Design review of the part built by this model. Coordinates are the model's own, in mm. A direction names the side the tool comes from. Give positions to 0.01 mm unless a question says otherwise; leave off trailing zeros. Loops run counter-clockwise (first coordinate to the right, second up) from the corner with the lowest first, then second, coordinate; pieces in that order, holes last. Notation, with made-up numbers: (-0.5, 4) - (46.5, 4) arc R23 cw to (46.5, 32) - close; hole circle Ø10 at (-36.5, 72.5). An arc over 180 degrees is marked (long way). One line per item, written item: value. Start each with the question number.
```python
from build123d import *

# Parameters (mm, degrees)
F0_W     = 46.54321
F0_H     = 54.078784
F1_DEPTH = 25.4
F2_R     = 6.959459
F2_R_2   = 6.442665
F3_DEPTH = 50.8
F4_R     = 2.356005
F5_DEPTH = 50.8


with BuildPart() as f1:
    # F0 (on Front) → F1 (new body)
    with BuildSketch(Plane.XZ):
        Rectangle(F0_W, F0_H)
    extrude(amount=F1_DEPTH)

    # F2 (on face) → F3 (cut)
    with BuildSketch(Plane.XY.offset(27.039392)):
        with Locations((-11.081717, -13.741329)):
            Circle(F2_R)
        with Locations((10.416814, -13.741329)):
            Circle(F2_R_2)
    extrude(amount=-F3_DEPTH, mode=Mode.SUBTRACT)

    # F4 (on face) → F5 (join)
    with BuildSketch(Plane.XZ.offset(25.4)):
        with Locations((0, 22.828339)):
            Circle(F4_R)
    extrude(amount=F5_DEPTH)


solid = f1.part
```
(1) Machinability: for faces 1 (the cylindrical face through (-12.59, -20.535, 1.995)), 2 (the flat face through (0, 0, 0)), 3 (the cylindrical face through (-0.307, -50.444, 25.164)), which of the approach directions +Z, -Z, +X, -X, +Y, -Y give a long, thin tool a straight path to every point of the face, cutting with its end or side? Answer none if there is none.
(2) Take a section at D-D on x = -6. State the section outline as (y, z) points.
(3) To check wall thickness, follow L1, parallel to X at y = -19, z = -8; L2, parallel to Y at x = 20.5, z = -5; L3, parallel to Y at x = 13, z = 0.5. State the ranges of each line that lie inside material, in increasing order. Write a range as from..to.
(4) Draft analysis for pull direction X (two halves, no side actions). For faces 4 (the flat face through (-23.272, -13, 0)), 5 (the flat face through (0, -76.2, 23)), 6 (the flat face through (10, -14, -23.761)), state which applies: pulls with the +X half, pulls with the -X half, needs draft (parallel to the pull), parting line crosses it, or undercut.
(5) For pin 1 Ø7 at (x, y) = (-13.5, -14) entering from +Z; pin 2 Ø14 at (x, z) = (8, -4) entering from -Y; pin 3 Ø12 at (x, y) = (9, -32) entering from +Z, all flat-tipped, find the tip position at first contact; note any pin that passes through.
(6) Take a section at B-B on z = 8.5. State the section outline as (x, y) points.
(7) Take a section at A-A on x = 0. State the section outline as (y, z) points.
(8) Take a section at C-C on y = -11. State the section outline as (x, z) points, and give its area (3 significant figures).
Here are the results:
1. face 1: +Z
1. face 2: +Z, -Z, +X, -X, +Y
1. face 3: -Y
2. outline: (-25.4, -27.04) - (0, -27.04) - (0, 27.04) - (-8.99, 27.04) - (-8.99, -23.76) - (-18.5, -23.76) - (-18.5, 27.04) - (-25.4, 27.04) - close
3. L1: -23.27..-15.64, -6.52..6.69, 14.14..23.27
3. L2: -25.4..0
3. L3: -25.4..-19.64, -7.84..0
4. face 4: pulls with the -X half
4. face 5: needs draft
4. face 6: undercut
5. pin 1: z = -23.76
5. pin 2: y = -25.4
5. pin 3: through
6. outline: (-23.27, -25.4) - (23.27, -25.4) - (23.27, 0) - (-23.27, 0) - close; hole circle Ø13.92 at (-11.08, -13.74); hole circle Ø12.89 at (10.42, -13.74)
7. outline: (-76.2, 20.47) - (-25.4, 20.47) - (-25.4, -27.04) - (0, -27.04) - (0, 27.04) - (-25.4, 27.04) - (-25.4, 25.18) - (-76.2, 25.18) - close
8. outline: (-23.27, -27.04) - (23.27, -27.04) - (23.27, 27.04) - (16.25, 27.04) - (16.25, -23.76) - (4.59, -23.76) - (4.59, 27.04) - (-4.68, 27.04) - (-4.68, -23.76) - (-17.48, -23.76) - (-17.48, 27.04) - (-23.27, 27.04) - close
8. area: 1,270 mm²
